Verification items for this drawing (mm, ordinates from the low corner). A direction names the side the tool comes from. Give positions to 0.01 mm unless a question says otherwise; leave off trailing zeros. Write each loop counter-clockwise with the first axis right and the second up, starting at its lowest first coordinate (ties: lowest second). Pieces come first, ordered by that corner, then holes. Notation, with made-up numbers: (60.25, 63.5) -> (94.25, 63.5) arc R11 ccw to (94.25, 70.5) -> close; hole circle Ø5 at (52.25, 73.25). An arc over 180 degrees is marked (long way). One line per item, written item: value.
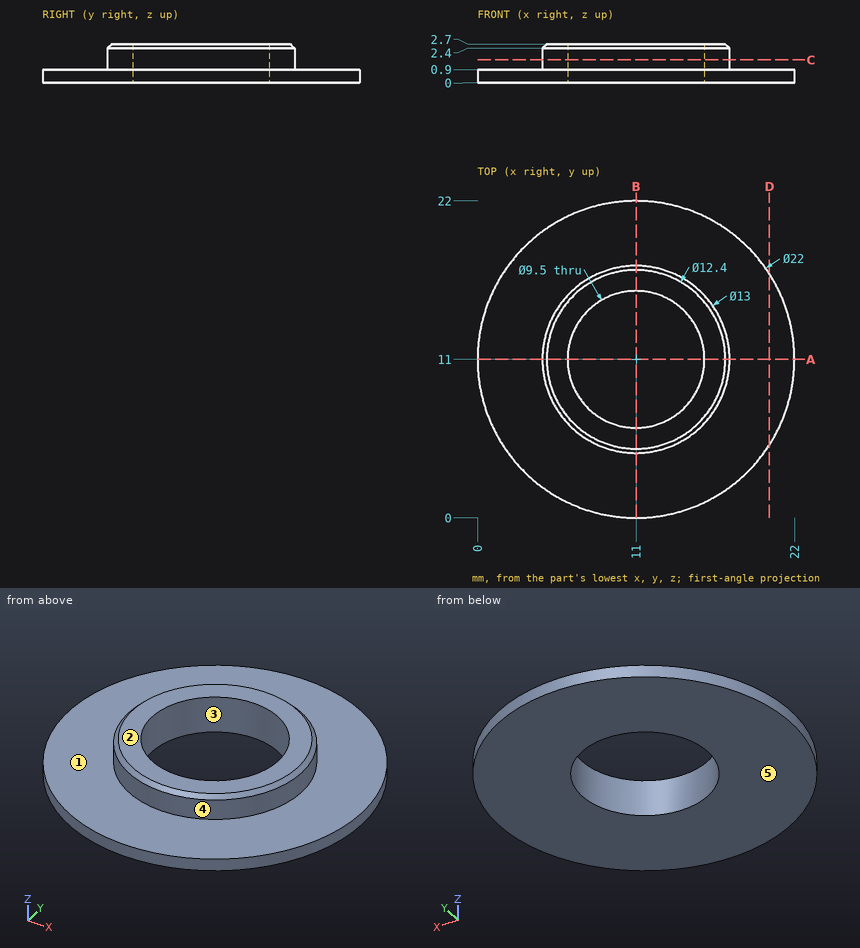
1) Scan lines: probe 1 along Y at (x, z) = (11, 1.1); probe 2 along Z at (x, y) = (10, 2.5); probe 3 along X at (y, z) = (7.5, 0.85). Record each from-to range of solid material in increasing order.
Verdict:
probe 1: 4.5 to 6.25, 15.75 to 17.5
probe 2: 0 to 0.9
probe 3: 0.57 to 7.79, 14.21 to 21.43
2) Depth check by flat-ended pin: pin 1 Ø2 at (x, y) = (9, 12.5) entering from +Z; pin 2 Ø1.5 at (x, z) = (17, 2) entering from -Y. Enter the tip coordinate at first touch or a pass-through.
Verdict:
pin 1: through
pin 2: y = 7.17
3) Mould release check, pull along Y, two halves, no side actions. Record for the marked faces 3, 4 and 5: released by +Y, released by -Y, zero draft, split by the parting line, or undercut.
Verdict:
face 3: undercut
face 4: split by the parting line
face 5: zero draft
4) Sectioned sample at D-D on x = 20.25. Record the cut outline in (y, z).
Verdict:
outline: (5.05, 0) -> (16.95, 0) -> (16.95, 0.9) -> (5.05, 0.9) -> close
5) Sectioned sample at C-C on z = 1.6. Record the cut outline in (x, y), plus the area to 4 significant figures.
Verdict:
outline: circle Ø13 at (11, 11); hole circle Ø9.5 at (11, 11)
area: 61.85 mm^2
6) Sectioned sample at A-A on y = 11. Record the cut outline in (x, z), plus the area to 3 significant figures.
Verdict:
outline: (0, 0) -> (6.25, 0) -> (6.25, 2.7) -> (4.8, 2.7) -> (4.5, 2.4) -> (4.5, 0.9) -> (0, 0.9) -> close; (15.75, 0) -> (22, 0) -> (22, 0.9) -> (17.5, 0.9) -> (17.5, 2.4) -> (17.2, 2.7) -> (15.75, 2.7) -> close
area: 17.5 mm^2
7) Tool access check on the marked faces 1 and 2. Record the directions out of +Z, -Z, +X, -X, +Y, -Y that give a thin tool (end or side, any length) a straight path to the whole face; none if there is none.
Verdict:
face 1: +Z
face 2: +Z, +X, -X, +Y, -Y
